Input: part model. Units: mm. Frame: model coordinates. Face numbers are marked on the shaded views. Give positions to 0.01 mm unless a question says otherwise; leave off trailing zeros. Write each loop counter-clockwise with the first axis right and the second up, starting at its lowest first coordinate (ties: lowest second). Pieces come first, ordered by that corner, then holes.
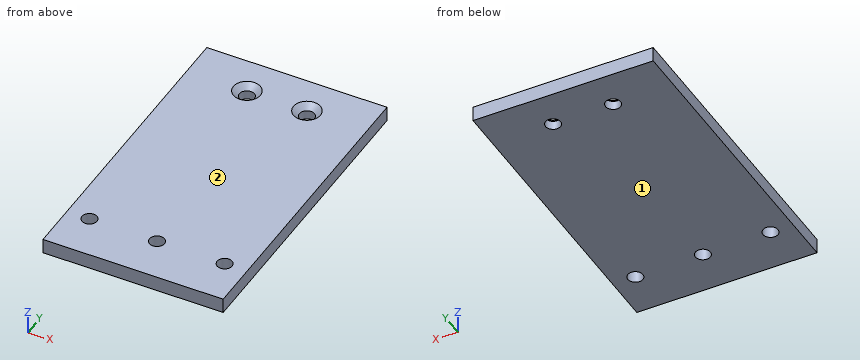
```python
from build123d import *

# Parameters (mm, degrees)
SKETCH1_W           = 76.2
SKETCH1_H           = 139.7
BOSS_EXTRUDE1_DEPTH = 6.35
SKETCH2_R           = 3.175
CUT_EXTRUDE1_DEPTH  = 6.35
CHAMFER2_SIZE       = 2.54
SKETCH3_W           = 6.35
SKETCH3_H           = 9.525
CUT_EXTRUDE2_DEPTH  = 104.565365832


with BuildPart() as part:
    # Sketch1 → Boss-Extrude1 (new body)
    with BuildSketch(Plane.XY):
        Rectangle(SKETCH1_W, SKETCH1_H)
    extrude(amount=BOSS_EXTRUDE1_DEPTH)

    # Sketch2 → Cut-Extrude1 (cut)
    with BuildSketch(Plane.XY.offset(6.35)):
        with Locations((-12.7, 44.45)):
            Circle(SKETCH2_R)
        with Locations((12.7, 44.45)):
            Circle(SKETCH2_R)
        with Locations((-28.575, -50.8)):
            Circle(SKETCH2_R)
        with Locations((0, -50.8)):
            Circle(SKETCH2_R)
        with Locations((28.575, -50.8)):
            Circle(SKETCH2_R)
    extrude(amount=-CUT_EXTRUDE1_DEPTH, mode=Mode.SUBTRACT)

    # Chamfer2
    chamfer2_edges = [part.edges().sort_by_distance(p)[0] for p in [
        (-15.875, 44.45, 6.35),
        (9.525, 44.45, 6.35),
    ]]
    chamfer(chamfer2_edges, length=CHAMFER2_SIZE)

    # Sketch3 → Cut-Extrude2 (cut, through all)
    with BuildSketch(Plane.ZY.offset(38.1)):
        with Locations((3.175, 65.0875)):
            Rectangle(SKETCH3_W, SKETCH3_H)
    extrude(amount=-CUT_EXTRUDE2_DEPTH, mode=Mode.SUBTRACT)


solid = part.part
```
Q1. Section D-D, the plane x = -12.7. Return the cut outline in (y, z) (3 decimals).
Q2. Section B-B, the plane y = 44.45. Return the cut outline in (x, z) (3 decimals), then the cut area to 3 significant figures.
Q3. Pin query (flat end, axial travel): pin 1 (10 mm diameter, centred on x = -12.7, y = 44.45, fed in from +Z) (3 decimals); pin 2 (4 mm diameter, centred on x = -28.575, y = -50.8, fed in from -Z). Return the tip coordinate at first contact, or that it passes through.
Q4. Material intervals for line 1 along Y through (x, z) = (-12.7, 1.35) (3 decimals); line 2 along Y through (x, z) = (0, 4) (3 decimals); line 3 along X through (y, z) = (42.5, 5.25), sorted ascending.
Q5. Mould query, pull axis Z, two halves, no side actions, for the marked faces 1 and 2. Classes: +Z half, -Z half, draft (parallel to the pull), parting line (faces both ways), or undercut.
Q6. Section C-C, the plane y = -50.8. Return the cut outline in (x, z) (3 decimals).
Q7. Section A-A, the plane x = 0. Return the cut outline in (y, z) (3 decimals), then the cut area to 3 significant figures.
Solutions:
1. outline: (-69.85, 0) - (41.275, 0) - (41.275, 3.81) - (38.735, 6.35) - (-69.85, 6.35) - close; (47.625, 0) - (60.325, 0) - (60.325, 6.35) - (50.165, 6.35) - (47.625, 3.81) - close
2. outline: (-38.1, 0) - (-15.875, 0) - (-15.875, 3.81) - (-18.415, 6.35) - (-38.1, 6.35) - close; (-9.525, 0) - (9.525, 0) - (9.525, 3.81) - (6.985, 6.35) - (-6.985, 6.35) - (-9.525, 3.81) - close; (15.875, 0) - (38.1, 0) - (38.1, 6.35) - (18.415, 6.35) - (15.875, 3.81) - close
2. area: 390 mm2
3. pin 1: stops at z = 5.635
3. pin 2: passes through
4. line 1: y = -69.85 to 41.275, 47.625 to 60.325
4. line 2: y = -69.85 to -53.975, -47.625 to 60.325
4. line 3: x = -38.1 to -16.88, -8.52 to 8.52, 16.88 to 38.1
5. face 1: -Z half
5. face 2: +Z half
6. outline: (-38.1, 0) - (-31.75, 0) - (-31.75, 6.35) - (-38.1, 6.35) - close; (-25.4, 0) - (-3.175, 0) - (-3.175, 6.35) - (-25.4, 6.35) - close; (3.175, 0) - (25.4, 0) - (25.4, 6.35) - (3.175, 6.35) - close; (31.75, 0) - (38.1, 0) - (38.1, 6.35) - (31.75, 6.35) - close
7. outline: (-69.85, 0) - (-53.975, 0) - (-53.975, 6.35) - (-69.85, 6.35) - close; (-47.625, 0) - (60.325, 0) - (60.325, 6.35) - (-47.625, 6.35) - close
7. area: 786 mm2
